The listing builds one solid part. Answer for the finished solid, in the listing's coordinates (mm). A direction names the side the tool comes from. Give positions to 0.01 mm unless a question says otherwise; leave off trailing zeros. Loops run counter-clockwise (first coordinate to the right, second up) from the corner with the lowest first, then second, coordinate; pieces in that order, holes last. Notation, with made-up numbers: (-2, -23) - (51, -23) arc R16 cw to (51, -19) - close; hole circle Ø4 at (88, 10). An arc over 180 degrees is marked (long way). Write each question's results on one line, items separated by ' | '.
Autodesk Inventor part; units mm, degrees
ref_plane "YZ Plane" through (0, 0, 0) normal (1, 0, 0) x (0, 1, 0)
ref_plane "XZ Plane" through (0, 0, 0) normal (0, 1, 0) x (-1, 0, 0)
ref_plane "XY Plane" through (0, 0, 0) normal (0, 0, 1) x (1, 0, 0)
sketch "Sketch1" plane through (0, 0, 0) normal (0, 1, 0) x (-1, 0, 0)
  circle A0 centre (0, 0) radius 2.5
  circle A1 centre (0, 0) radius 9
  circle A2 centre (0, 0) radius 6
  dimension "d0" = 5
  dimension "d1" = 18
  dimension "d2" = 12
extrude "Extrusion1" add sketch "Sketch1" along normal blind 11 contours A2
extrude "Extrusion2" add sketch "Sketch1" along normal blind 1 from surface at 11 contours A1 | A2
extrude "Extrusion3" add sketch "Sketch1" against normal blind 1 contours A1 | A2
properties part number "Idler"
Item 1: A cutting plane is placed at C-C, the plane z = -4.25. Determine the outline of the cut face in (x, y), plus the area to 3 significant figures.
Values found:
outline: (-7.93, -1) - (7.93, -1) - (7.93, 0) - (4.24, 0) - (4.24, 11) - (7.93, 11) - (7.93, 12) - (-7.93, 12) - (-7.93, 11) - (-4.24, 11) - (-4.24, 0) - (-7.93, 0) - close | area: 125 mm²
Item 2: Find the intervals of material crossed by line 1 along Z through (x, y) = (0, 6.25); line 2 along Y through (x, z) = (7, 0.25); line 3 along X through (y, z) = (4, 2), in increasing order. Write a range as [from, to].
Values found:
line 1: z = [-6, -2.5], [2.5, 6] | line 2: y = [-1, 0], [11, 12] | line 3: x = [-5.66, -1.5], [1.5, 5.66]
Item 3: For faces 1 (the face through (0.54, 5.41, 2.44)), 2 (the face through (-2, 0, -6)), determine the directions among +Z, -Z, +X, -X, +Y, -Y from which every point of the face is accessible in a straight line to the end or side of a thin tool.
Values found:
face 1: +Y, -Y | face 2: none
Item 4: A cutting plane is placed at D-D, the plane y = 9. Determine the outline of the cut face in (x, z), plus the area to 3 significant figures.
Values found:
outline: circle Ø12 at (0, 0); hole circle Ø5 at (0, 0) | area: 93.5 mm²
Item 5: For a pull along Y with two mould halves and no side action, classify faces 3 (the face through (1.172, -0.493, 8.923)), 4 (the face through (-2, 12, -2)), 5 (the face through (-2, 11, -6)) as released by +Y, released by -Y, zero draft, split by the parting line, or undercut.
Values found:
face 3: zero draft | face 4: released by +Y | face 5: undercut
Item 6: A cutting plane is placed at B-B, the plane x = 0. Determine the outline of the cut face in (y, z).
Values found:
outline: (-1, -9) - (0, -9) - (0, -6) - (11, -6) - (11, -9) - (12, -9) - (12, -2.5) - (-1, -2.5) - close; (-1, 2.5) - (12, 2.5) - (12, 9) - (11, 9) - (11, 6) - (0, 6) - (0, 9) - (-1, 9) - close
Item 7: Flat-ended cylindrical pins translate along their axes: P1, Ø1.5, axis at x = 0, y = 5, coming from the -Z side; P2, Ø1.5, axis at x = -2.5, y = 3, coming from the +Z side; P3, Ø5, axis at x = -3, y = 2, coming from the -Z side. Find the tip coordinate at first contact, or state that the pin passes through.
Values found:
P1: stops at z = -6 | P2: stops at z = 5.74 | P3: stops at z = -8.87
Item 8: A cutting plane is placed at A-A, the plane z = 0. Determine the outline of the cut face in (x, y).
Values found:
outline: (-9, -1) - (-2.5, -1) - (-2.5, 12) - (-9, 12) - (-9, 11) - (-6, 11) - (-6, 0) - (-9, 0) - close; (2.5, -1) - (9, -1) - (9, 0) - (6, 0) - (6, 11) - (9, 11) - (9, 12) - (2.5, 12) - close
